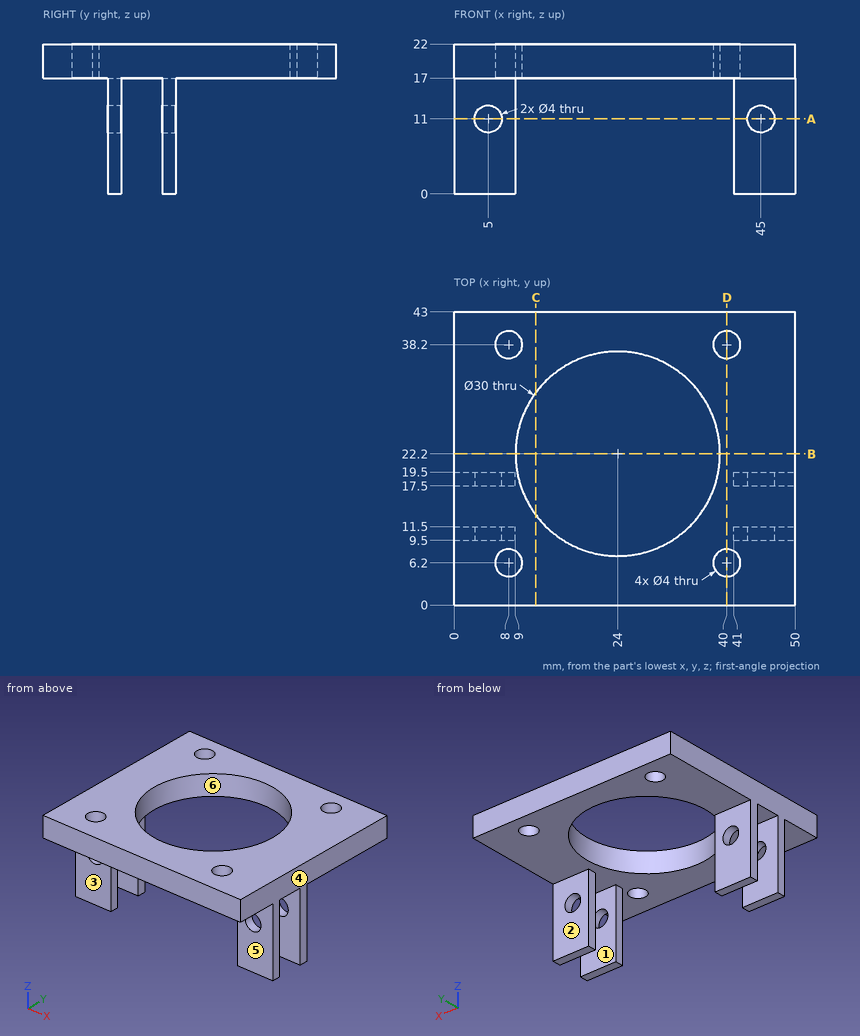
Study the drawing (mm; zero at the part's minimum x, y, z) and answer. A direction names the side the tool comes from. Give positions to 0.01 mm unless a question says otherwise; leave off trailing zeros. Write each loop counter-clockwise with the first axis right and the second up, starting at its lowest first coordinate (ties: lowest second). Pieces come first, ordered by that corner, then holes.
Item 1: Determine the mould class of the marked faces 4, 5 and 6 for opening direction X: released by +X, released by -X, zero draft, split by the parting line, or undercut.
Item 2: Flat-ended cylindrical pins translate along their axes: P1, Ø4.5, axis at x = 5, z = 10.5, coming from the +Y side; P2, Ø4.5, axis at x = 47.5, z = 12.5, coming from the -Y side; P3, Ø6.5, axis at x = 40, y = 38.2, coming from the -Z side. Find the tip coordinate at first contact, or state that the pin passes through.
Item 3: Section C-C, the plane x = 12 is taken. Write down the section's boundary in (y, z), plus the area to 3 significant figures.
Item 4: Find the intervals of material crossed by line 1 along Y through (x, z) = (40, 18.05); line 2 along Y through (x, z) = (48, 10); line 3 along Z through (x, y) = (5, 10.75), in increasing order.
Item 5: Section D-D, the plane x = 40 is taken. Write down the section's boundary in (y, z).
Item 6: Section B-B, the plane y = 22.2 is taken. Write down the section's boundary in (x, z), plus the area to 3 significant figures.
Item 7: Section A-A, the plane z = 11 is taken. Count the separate pieces of the cut face and the enclosed holes in it, plus the area to 3 significant figures.
Item 8: Which of the six approach directions +Z, -Z, +X, -X, +Y, -Y give full straight-line access (tool end or side, diameter ignored) to the marked faces 1, 2 and 3?
Completed:
1. face 4: released by +X
1. face 5: zero draft
1. face 6: undercut
2. P1: stops at y = 19.5
2. P2: stops at y = 9.5
2. P3: stops at z = 17
3. outline: (0, 17) - (13.2, 17) - (13.2, 22) - (0, 22) - close; (31.2, 17) - (43, 17) - (43, 22) - (31.2, 22) - close
3. area: 125 mm2
4. line 1: y = 0 to 4.2, 8.2 to 36.2, 40.2 to 43
4. line 2: y = 9.5 to 11.5, 17.5 to 19.5
4. line 3: z = 0 to 9, 13 to 22
5. outline: (0, 17) - (4.2, 17) - (4.2, 22) - (0, 22) - close; (8.2, 17) - (36.2, 17) - (36.2, 22) - (8.2, 22) - close; (40.2, 17) - (43, 17) - (43, 22) - (40.2, 22) - close
6. outline: (0, 17) - (9, 17) - (9, 22) - (0, 22) - close; (39, 17) - (50, 17) - (50, 22) - (39, 22) - close
6. area: 100 mm2
7. separate pieces: 8
7. enclosed holes: 0
7. area: 40.0 mm2
8. face 1: -Z, +X, -X
8. face 2: -Z, +X, -X, +Y
8. face 3: -Z, +X, -X, -Y
